Check sheet for the modelled part. Datum: model origin and axes. Units: mm. A direction names the side the tool comes from. Give positions to 0.01 mm unless a question says otherwise; leave off trailing zeros. Write each loop counter-clockwise with the first axis right and the second up, starting at its lowest first coordinate (ties: lowest second). Pieces come first, ordered by that corner, then holes. Notation, with made-up numbers: (-21.75, 77.5) -> (11.25, 77.5) arc R25 ccw to (11.25, 95.5) -> close; hole circle Ø11 at (-13, 33.5). An arc over 180 degrees is marked (long way). Answer as a JSON object with one key per item and string values.
from build123d import *

# Parameters (mm, degrees)
SKETCH1_W           = 58
SKETCH1_H           = 30
SKETCH1_R           = 3
BOSS_EXTRUDE1_DEPTH = 8
SKETCH2_W           = 26
SKETCH2_H           = 30
BOSS_EXTRUDE2_DEPTH = 8
SKETCH3_R           = 4
CUT_EXTRUDE1_DEPTH  = 37.359317925
CHAMFER1_SIZE       = 3


with BuildPart() as part:
    # Sketch1 → Boss-Extrude1 (new body)
    with BuildSketch(Plane(origin=(0, 0, 0), x_dir=(1, 0, 0), z_dir=(0, 1, 0))):
        Rectangle(SKETCH1_W, SKETCH1_H)
        with Locations(Location((-20, 0, 0), (0, 0, 270))):
            Circle(SKETCH1_R, mode=Mode.SUBTRACT)
        with Locations(Location((20, 0, 0), (0, 0, 270))):
            Circle(SKETCH1_R, mode=Mode.SUBTRACT)
    extrude(amount=BOSS_EXTRUDE1_DEPTH)

    # Sketch2 → Boss-Extrude2 (add)
    with BuildSketch(Plane(origin=(0, 8, 0), x_dir=(1, 0, 0), z_dir=(0, 1, 0))):
        Rectangle(SKETCH2_W, SKETCH2_H)
    extrude(amount=BOSS_EXTRUDE2_DEPTH)

    # Sketch3 → Cut-Extrude1 (cut, through all)
    with BuildSketch(Plane(origin=(0, 16, 0), x_dir=(1, 0, 0), z_dir=(0, 1, 0))):
        with Locations(Location((0, 0, 0), (0, 0, 270))):
            Circle(SKETCH3_R)
    extrude(amount=-CUT_EXTRUDE1_DEPTH, mode=Mode.SUBTRACT)

    # Chamfer1
    chamfer1_edges = [part.edges().sort_by_distance(p)[0] for p in [
        (29, 4, 15),
        (-29, 4, 15),
        (-29, 4, -15),
        (29, 4, -15),
    ]]
    chamfer(chamfer1_edges, length=CHAMFER1_SIZE)


solid = part.part
1. Access from +Z, -Z, +X, -X, +Y, -Y to the whole of each face (thin tool, end or side, straight path). Record for faces 1 (the face through (21, 8, -4)), 2 (the face through (-13, 12, 0)), 3 (the face through (28, 4, 13)).
Determined:
{"face 1": "+Z, -Z, +X, +Y", "face 2": "+Z, -Z, -X, +Y", "face 3": "+Z, +X, +Y, -Y"}
2. Mould release check, pull along Z, two halves, no side actions. Record for faces 4 (the face through (-22.93, 3.94, -0.65)), 5 (the face through (-27, 4, -14)), 6 (the face through (6, 0, 0)): released by +Z, released by -Z, zero draft, split by the parting line, or undercut.
Determined:
{"face 4": "undercut", "face 5": "released by -Z", "face 6": "zero draft"}
3. Sectioned sample at D-D, the plane z = 9. Enter the section's corners in (x, y).
Determined:
{"outline": "(-29, 0) -> (29, 0) -> (29, 8) -> (13, 8) -> (13, 16) -> (-13, 16) -> (-13, 8) -> (-29, 8) -> close"}
4. Go/stop test with flat-tipped pins: P1, Ø1.5, axis at x = -7, z = -3, coming from the -Y side; P2, Ø17.5, axis at x = -23, z = -4, coming from the +Y side; P3, Ø2.5, axis at y = 13, z = -3, coming from the +X side. Record where each tip stops, or that it passes through.
Determined:
{"P1": "y = 0", "P2": "y = 8", "P3": "x = 13"}
5. Sectioned sample at A-A, the plane x = -20. Enter the section's corners in (y, z).
Determined:
{"outline": "(0, -15) -> (8, -15) -> (8, -3) -> (0, -3) -> close; (0, 3) -> (8, 3) -> (8, 15) -> (0, 15) -> close"}
6. Sectioned sample at C-C, the plane z = 0. Enter the section's corners in (x, y).
Determined:
{"outline": "(-29, 0) -> (-23, 0) -> (-23, 8) -> (-29, 8) -> close; (-17, 0) -> (-4, 0) -> (-4, 16) -> (-13, 16) -> (-13, 8) -> (-17, 8) -> close; (4, 0) -> (17, 0) -> (17, 8) -> (13, 8) -> (13, 16) -> (4, 16) -> close; (23, 0) -> (29, 0) -> (29, 8) -> (23, 8) -> close"}
7. Sectioned sample at B-B, the plane y = 4. Enter the section's corners in (x, z).
Determined:
{"outline": "(-29, -12) -> (-26, -15) -> (26, -15) -> (29, -12) -> (29, 12) -> (26, 15) -> (-26, 15) -> (-29, 12) -> close; hole circle Ø6 at (-20, 0); hole circle Ø8 at (0, 0); hole circle Ø6 at (20, 0)"}
8. Scan lines: L1, parallel to X at y = 6.5, z = 0; L2, parallel to X at y = 2.5, z = -2; L3, parallel to X at y = 13.75, z = 11. Record each from-to range of solid material in increasing order. Write a range as [from, to].
Determined:
{"L1": "[-29, -23], [-17, -4], [4, 17], [23, 29]", "L2": "[-29, -22.24], [-17.76, -3.46], [3.46, 17.76], [22.24, 29]", "L3": "[-13, 13]"}
